from build123d import *

# Parameters (mm, degrees)
SKETCH1_W           = 101
SKETCH1_H           = 110
BOSS_EXTRUDE1_DEPTH = 2
SKETCH3_W           = 15
SKETCH3_H           = 1.5
SKETCH3_W_2         = 3
SKETCH3_H_2         = 15
CUT_EXTRUDE1_DEPTH  = 128.433943673
SKETCH4_R           = 1.75
BOSS_EXTRUDE2_DEPTH = 5
SKETCH5_R           = 4
BOSS_EXTRUDE3_DEPTH = 2
FILLET1_R           = 0.5
FILLET2_R           = 25
SKETCH6_W           = 40
SKETCH6_H           = 3
BOSS_EXTRUDE4_DEPTH = 1
BOSS_EXTRUDE5_DEPTH = 40
SKETCH9_W           = 26
SKETCH9_H           = 75
CUT_EXTRUDE2_DEPTH  = 128.516312682
FILLET3_R           = 5


with BuildPart() as part:
    # Sketch1 → Boss-Extrude1 (new body)
    with BuildSketch(Plane.XY):
        with Locations((42.5, 32.1)):
            Rectangle(SKETCH1_W, SKETCH1_H)
    extrude(amount=BOSS_EXTRUDE1_DEPTH)

    # Sketch3 → Cut-Extrude1 (cut, through all)
    with BuildSketch(Plane.XY.offset(2)):
        with Locations((42.5, 81.35)):
            Rectangle(SKETCH3_W, SKETCH3_H)
        with Locations((-1.5, 19.1)):
            Rectangle(SKETCH3_W_2, SKETCH3_H_2)
        with Locations((86.5, 19.1)):
            Rectangle(SKETCH3_W_2, SKETCH3_H_2)
    extrude(amount=-CUT_EXTRUDE1_DEPTH, mode=Mode.SUBTRACT)

    # Sketch4 → Boss-Extrude2 (add)
    with BuildSketch(Plane.XY.offset(2)):
        with Locations((22.5, 27.1)):
            Circle(SKETCH4_R)
        with Locations((62.5, 27.1)):
            Circle(SKETCH4_R)
    extrude(amount=BOSS_EXTRUDE2_DEPTH)

    # Sketch5 → Boss-Extrude3 (add)
    with BuildSketch(Plane.XY.offset(7)):
        with Locations((22.5, 27.1)):
            Circle(SKETCH5_R)
        with Locations((62.5, 27.1)):
            Circle(SKETCH5_R)
    extrude(amount=-BOSS_EXTRUDE3_DEPTH)

    # Fillet1
    fillet1_edges = [part.edges().sort_by_distance(p)[0] for p in [
        (18.5, 27.1, 5),
        (18.5, 27.1, 7),
        (58.5, 27.1, 5),
        (58.5, 27.1, 7),
    ]]
    fillet(fillet1_edges, radius=FILLET1_R)

    # Fillet2
    fillet2_edges = [part.edges().sort_by_distance(p)[0] for p in [
        (-8, 87.1, 1),
        (93, 87.1, 1),
        (93, -22.9, 1),
        (-8, -22.9, 1),
    ]]
    fillet(fillet2_edges, radius=FILLET2_R)

    # Sketch6 → Boss-Extrude4 (add)
    with BuildSketch(Plane.XY.offset(2)):
        with Locations((42.5, -16.15)):
            Rectangle(SKETCH6_W, SKETCH6_H)
    extrude(amount=BOSS_EXTRUDE4_DEPTH)

    # Sketch7 → Boss-Extrude5 (add)
    with BuildSketch(Plane(origin=(62.5, 0, 0), x_dir=(0, 0, -1), z_dir=(1, 0, 0))):
        with BuildLine():
            Line((-3, -14.65), (-3, -17.65))
            ThreePointArc((-3, -17.65), (-4, -16.15), (-3, -14.65))
        make_face()
    extrude(amount=-BOSS_EXTRUDE5_DEPTH)

    # Sketch9 → Cut-Extrude2 (cut, through all)
    with BuildSketch(Plane.XY.offset(2)):
        with Locations((42.5, 30.6)):
            Rectangle(SKETCH9_W, SKETCH9_H)
    extrude(amount=-CUT_EXTRUDE2_DEPTH, mode=Mode.SUBTRACT)

    # Fillet3
    fillet3_edges = [part.edges().sort_by_distance(p)[0] for p in [
        (29.5, -6.9, 1),
        (29.5, 68.1, 1),
        (55.5, 68.1, 1),
        (55.5, -6.9, 1),
    ]]
    fillet(fillet3_edges, radius=FILLET3_R)


solid = part.part
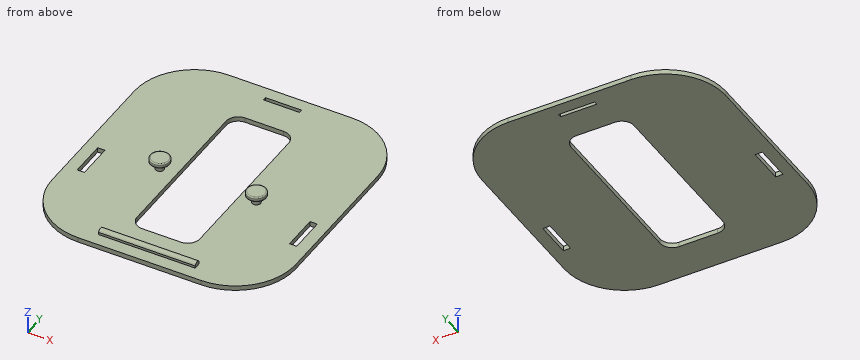
The model under review builds one solid part; all positions refer to its coordinate system, in mm. Round coordinates to 2 decimals unless told otherwise and drop trailing zeros. Order: outer loops, then holes, each group sorted by start corner. A loop starts at its lowest first (then second) coordinate and runs counter-clockwise, first axis right, second up. Notation, with made-up numbers: (-21.75, -21.75) -> (16.25, -21.75) arc R11 ccw to (16.25, -9.75) -> close; hole circle Ø7 at (86.25, 47). An arc over 180 degrees is marked (long way). Write item = value, one per line. Start each with the question number.
Item 1: For line 1 along Y through (x, z) = (41, 1.75); line 2 along X through (y, z) = (26, 1); line 3 along X through (y, z) = (61, 1.75), list the stretches that pass through material, from the lowest coordinate up.
Item 2: Consider section A-A on y = 19. Write out the cut boundary in (x, z).
Item 3: Consider section B-B on y = 49.5. Write out the cut boundary in (x, z).
Item 4: Clearance check with flat-ended pins moving along their axes: pin 1 Ø12 at (x, y) = (38, 50.5) entering from -Z; pin 2 Ø0.5 at (x, z) = (48.5, 2.5) entering from -Y; pin 3 Ø0.6 at (x, z) = (-1, 1) entering from +Y; pin 4 Ø0.8 at (y, z) = (81, 1) entering from -X. State where each tip first meets the part, or that it passes through.
Item 5: Consider section D-D on y = 76.5. Write out the cut boundary in (x, z), plus the area to 3 significant figures.
Item 6: Consider section C-C on x = 81. Write out the cut boundary in (y, z), plus the area to 3 significant figures.
Conclusion:
q1.line_1 = -22.9 to -6.9, 68.1 to 80.6, 82.1 to 87.1
q1.line_2 = -8 to -3, 0 to 29.5, 55.5 to 85, 88 to 93
q1.line_3 = -8 to 29.5, 55.5 to 93
q2.outline = (-8, 0) -> (-3, 0) -> (-3, 2) -> (-8, 2) -> close; (0, 0) -> (29.5, 0) -> (29.5, 2) -> (0, 2) -> close; (55.5, 0) -> (85, 0) -> (85, 2) -> (55.5, 2) -> close; (88, 0) -> (93, 0) -> (93, 2) -> (88, 2) -> close
q3.outline = (-8, 0) -> (29.5, 0) -> (29.5, 2) -> (-8, 2) -> close; (55.5, 0) -> (93, 0) -> (93, 2) -> (55.5, 2) -> close
q4.pin_1 = through
q4.pin_2 = -17.65
q4.pin_3 = 79.76
q4.pin_4 = 0.18
q5.outline = (-3.44, 0) -> (88.44, 0) -> (88.44, 2) -> (-3.44, 2) -> close
q5.area = 184 mm2
q6.outline = (-19.25, 0) -> (83.45, 0) -> (83.45, 2) -> (-19.25, 2) -> close
q6.area = 205 mm2
